from build123d import *

# Parameters (mm, degrees)
SKETCH_1_W          = 110
SKETCH_1_H          = 78
SKETCH_1_R          = 1.6
EXTRUDE_1_DEPTH     = 3
FILLET_1_R          = 3
SKETCH_2_R          = 1.5
CUT_EXTRUDE_1_DEPTH = 10


with BuildPart() as part:
    # 草图1 → 凸台-拉伸1 (new body)
    with BuildSketch(Plane(origin=(0, 0, 0), x_dir=(1, 0, 0), z_dir=(0, 1, 0))):
        Rectangle(SKETCH_1_W, SKETCH_1_H)
        with Locations(Location((-37, 36, 0), (0, 0, 270))):
            Circle(SKETCH_1_R, mode=Mode.SUBTRACT)
        with Locations(Location((37, 36, 0), (0, 0, 270))):
            Circle(SKETCH_1_R, mode=Mode.SUBTRACT)
        with Locations(Location((37, -36, 0), (0, 0, 270))):
            Circle(SKETCH_1_R, mode=Mode.SUBTRACT)
        with Locations(Location((-37, -36, 0), (0, 0, 270))):
            Circle(SKETCH_1_R, mode=Mode.SUBTRACT)
    extrude(amount=EXTRUDE_1_DEPTH)

    # 圆角1
    fillet_1_edges = [part.edges().sort_by_distance(p)[0] for p in [
        (-55, 1.5, -39),
        (55, 1.5, -39),
        (55, 1.5, 39),
        (-55, 1.5, 39),
    ]]
    fillet(fillet_1_edges, radius=FILLET_1_R)

    # 草图2 → 切除-拉伸1 (cut)
    with BuildSketch(Plane(origin=(0, 3, 0), x_dir=(1, 0, 0), z_dir=(0, 1, 0))):
        with Locations(Location((0, 7, 0), (0, 0, 270))):
            Circle(SKETCH_2_R)
        with Locations(Location((7, 0, 0), (0, 0, 270))):
            Circle(SKETCH_2_R)
        with Locations(Location((0, -7, 0), (0, 0, 270))):
            Circle(SKETCH_2_R)
        with Locations(Location((-7, 0, 0), (0, 0, 270))):
            Circle(SKETCH_2_R)
        with Locations(Location((18.6, 0, 0), (0, 0, 270))):
            Circle(SKETCH_2_R)
        with Locations(Location((-18.6, 0, 0), (0, 0, 270))):
            Circle(SKETCH_2_R)
        with Locations(Location((0, 18.6, 0), (0, 0, 270))):
            Circle(SKETCH_2_R)
        with Locations(Location((0, -18.6, 0), (0, 0, 270))):
            Circle(SKETCH_2_R)
    extrude(amount=-CUT_EXTRUDE_1_DEPTH, mode=Mode.SUBTRACT)


solid = part.part
Verification items for the finished model (mm, model axes). Give positions to 0.01 mm unless a question says otherwise; leave off trailing zeros. Order: outer loops, then holes, each group sorted by start corner. A loop starts at its lowest first (then second) coordinate and runs counter-clockwise, first axis right, second up. Notation, with made-up numbers: M 44,57 L 77,57 A22 ccw 77,87 Z; hole C 47.5,40.25 d9. An arc over 180 degrees is marked long. Answer as a JSON object with one key per item and string values. Group by question number.
1) Mould release check, pull along Z, two halves, no side actions. Record for faces 1 (the face through (-1, 1, 39)), 2 (the face through (-8.464, 1.521, -0.325)), 3 (the face through (55, 1, 1)): released by +Z, released by -Z, zero draft, split by the parting line, or undercut.
2) Cross-section at B-B (x = 37). Enter the section's corners in (y, z).
3) Cross-section at C-C (z = -18.6). Enter the section's corners in (x, y), then the cut area to 3 significant figures.
4) Scan lines: line 1 along X through (y, z) = (2, -36); line 2 along X through (y, z) = (2.1, 0); line 3 along Z through (x, y) = (-1, 1.65). Record each from-to range of solid material in increasing order. Write a range as [from, to].
5) Depth check by flat-ended pin: pin 1 Ø8 at (x, z) = (32, 8) entering from -Y. Enter the tip coordinate at first touch or a pass-through.
6) Cross-section at A-A (x = 7). Enter the section's corners in (y, z).
Result sheet:
{
 "1": {"face 1": "released by +Z", "face 2": "undercut", "face 3": "zero draft"},
 "2": {"outline": "M 0,-39 L 3,-39 L 3,-37.6 L 0,-37.6 Z; M 0,-34.4 L 3,-34.4 L 3,34.4 L 0,34.4 Z; M 0,37.6 L 3,37.6 L 3,39 L 0,39 Z"},
 "3": {"outline": "M -55,0 L -1.5,0 L -1.5,3 L -55,3 Z; M 1.5,0 L 55,0 L 55,3 L 1.5,3 Z", "area": "321 mm2"},
 "4": {"line 1": "x = [-55, -38.6], [-35.4, 35.4], [38.6, 55]", "line 2": "x = [-55, -20.1], [-17.1, -8.5], [-5.5, 5.5], [8.5, 17.1], [20.1, 55]", "line 3": "z = [-39, -19.72], [-17.48, -8.12], [-5.88, 5.88], [8.12, 17.48], [19.72, 39]"},
 "5": {"pin 1": "stops at y = 0"},
 "6": {"outline": "M 0,-39 L 3,-39 L 3,-1.5 L 0,-1.5 Z; M 0,1.5 L 3,1.5 L 3,39 L 0,39 Z"}
}
